The listing builds one solid part. Answer for the finished solid, in the listing's coordinates (mm). A direction names the side the tool comes from. Round coordinates to 2 decimals unless told otherwise and drop trailing zeros. Loops run counter-clockwise (first coordinate to the right, second up) from the corner with the lowest first, then second, coordinate; pieces in that order, holes last. Notation, with made-up numbers: (5.25, 70.25) - (24.25, 70.25) arc R22 cw to (24.25, 76.25) - close; hole circle Ø10 at (-1, 80). An arc over 180 degrees is marked (long way). Write item = value, one per line. Start each with the question number.
1) Given pin 1 Ø5 at (x, z) = (9, -3.5) entering from -Y; pin 2 Ø1 at (x, y) = (33, -2) entering from +Z; pin 3 Ø6 at (x, z) = (26.5, -1.5) entering from -Y, each flat-ended and moving along its own axis, determine where each tip first touches the part or whether it passes through.
2) Section A-A, the plane x = 14 is taken. Determine the outline of the cut face in (y, z), and give its area (3 significant figures).
3) A tool of negligible diameter and unlimited length cuts with its end or side. For faces 1 (the cylindrical face through (28.63, -1.08, -4.88)), 2 (the flat face through (3.377, -6.896, -4.056)), from which of +Z, -Z, +X, -X, +Y, -Y can it reach the whole face along a straight path? Write none if from no direction.
4) Straight lines are drawn through the part: line 1 along X through (y, z) = (-6, -1.25); line 2 along Y through (x, z) = (36, -0.75). For each, find the intervals that lie inside material, in ascending order.
5) For a pull along Z with two mould halves and no side action, classify faces 3 (the conical face through (0.174, 8.301, -0.02)), 4 (the flat face through (3, 0, 8)), 5 (the flat face through (6.85, -4, 3.4)) as released by +Z, released by -Z, zero draft, split by the parting line, or undercut.
from build123d import *

# Parameters (mm, degrees)
BASEHEAD_DEPTH = 6.85


with BuildPart() as part:
    # Sketch1 → BaseHead (new body)
    with BuildSketch(Plane(origin=(0, 0, 0), x_dir=(0, 0, -1), z_dir=(1, 0, 0))):
        Polygon((8, 4.618802154), (8, -4.618802154), (0, -9.237604307), (-8, -4.618802154), (-8, 4.618802154), (0, 9.237604307), align=None)
    extrude(amount=BASEHEAD_DEPTH)

    # BodySke → BaseBody (revolve)
    with BuildSketch(Plane.XY):
        Polygon((0, 0), (51.85, 0), (51.85, 4.172), (51.022, 5), (0, 5), align=None)
    revolve(axis=Axis((0, 0, 0), (1, 0, 0)))

    # Sketch3 → HeadChamfer (revolve, cut)
    with BuildSketch(Plane.XY):
        Polygon((0, 8), (3.601282526, 14.237604307), (3.601282526, 19.237604307), (-10, 19.237604307), (-10, 8), align=None)
    revolve(axis=Axis((0, 0, 0), (1, 0, 0)), mode=Mode.SUBTRACT)


solid = part.part
Geometry check:
q1.pin_1 = -7.95
q1.pin_2 = 4.77
q1.pin_3 = -5
q2.outline = circle Ø10 at (0, 0)
q2.area = 78.5 mm2
q3.face_1 = +X
q3.face_2 = -Z, +X, -X, -Y
q4.line_1 = 0 to 6.85
q4.line_2 = -4.94 to 4.94
q5.face_3 = split by the parting line
q5.face_4 = released by +Z
q5.face_5 = zero draft
